Check sheet for the drawn part. Datum: minimum x, y, z corner. Units: mm. A direction names the side the tool comes from. Give positions to 0.01 mm unless a question says otherwise; leave off trailing zeros. Order: outer loops, then holes, each group sorted by start corner. A loop starts at its lowest first (then second) coordinate and runs counter-clockwise, first axis right, second up. Notation, with made-up numbers: (73.5, 21) - (114.5, 21) arc R27 ccw to (114.5, 57) - close; hole circle Ø2 at (46.25, 85.25). An arc over 180 degrees is marked (long way). Answer as a JSON object with one key per item and string values. Group by question number.
(1) Depth check by flat-ended pin: pin 1 Ø4.5 at (x, y) = (19.5, 3) entering from -Z; pin 2 Ø1.5 at (x, z) = (13, 29) entering from +Y; pin 3 Ø1 at (y, z) = (1, 24.5) entering from +X. Enter the tip coordinate at first touch or a pass-through.
(2) Section check B-B (x = 7.5). Record the boundary of the cut face in (y, z), then the cut area to 3 significant figures.
(3) Access from +Z, -Z, +X, -X, +Y, -Y to the whole of each face (thin tool, end or side, straight path). Record for the marked faces 4, 5 and 6.
(4) Thickness scan on line 1 (Z direction, x = 7.5, y = 0.95); line 2 (X direction, y = 1.45, z = 8); line 3 (Z direction, x = 16.75, y = 7). Record the ranges inside material, lowest first.
(5) Mould release check, pull along Z, two halves, no side actions. Record for the marked faces 1, 2 and 3: +Z half, -Z half, draft (parallel to the pull), parting line (faces both ways), or undercut.
(6) Section check A-A (z = 33). Record the boundary of the cut face in (x, y), then the cut area to 3 significant figures.
(7) Section check C-C (y = 8.5). Record the boundary of the cut face in (x, z).
(8) Section check D-D (z = 15). Record the boundary of the cut face in (x, y).
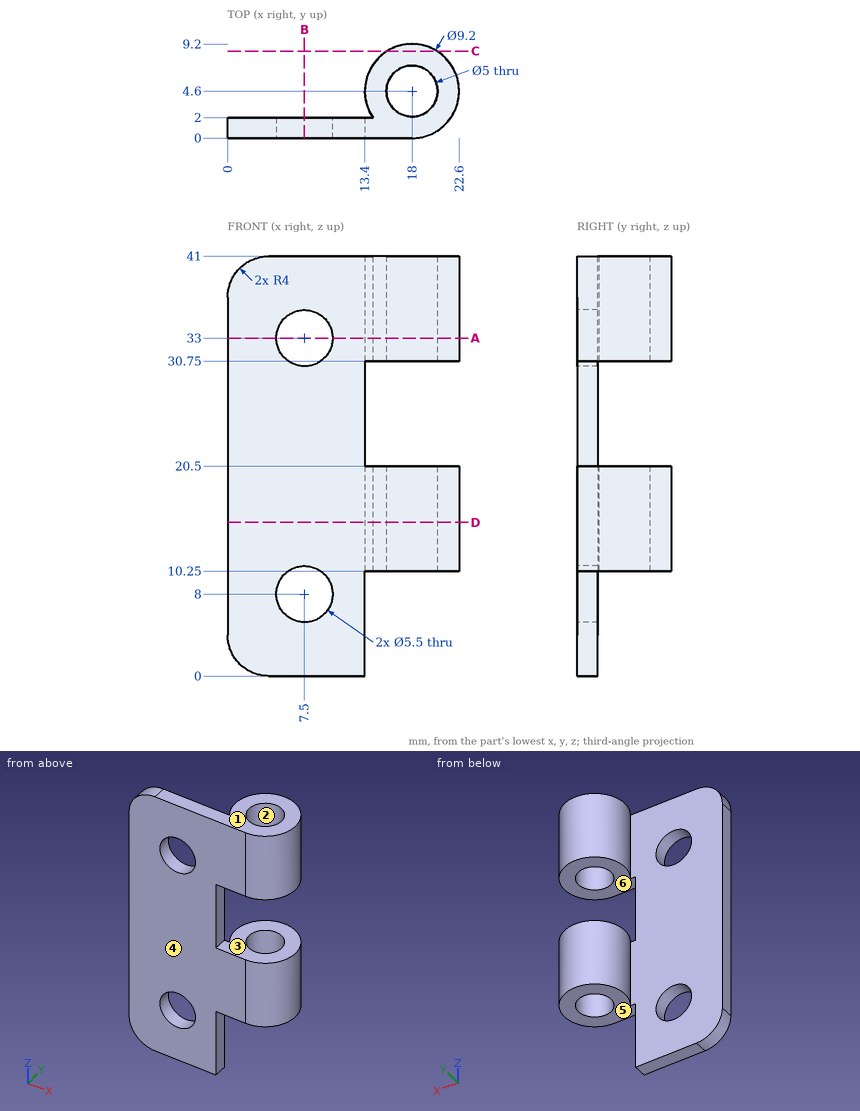
Solutions:
{
 "1": {"pin 1": "stops at z = 10.25", "pin 2": "stops at y = 2", "pin 3": "stops at x = 13.4"},
 "2": {"outline": "(0, 0) - (2, 0) - (2, 5.25) - (0, 5.25) - close; (0, 10.75) - (2, 10.75) - (2, 30.25) - (0, 30.25) - close; (0, 35.75) - (2, 35.75) - (2, 41) - (0, 41) - close", "area": "60.0 mm2"},
 "3": {"face 4": "+Z, -Z, +X, -X, -Y", "face 5": "-Z, +X, +Y, -Y", "face 6": "+X, +Y, -Y"},
 "4": {"line 1": "z = 0 to 5.25, 10.75 to 30.25, 35.75 to 41", "line 2": "x = 0 to 4.75, 10.25 to 13.4", "line 3": "z = 10.25 to 20.5, 30.75 to 41"},
 "5": {"face 1": "+Z half", "face 2": "draft", "face 3": "undercut"},
 "6": {"outline": "(0, 0) - (4.75, 0) - (4.75, 2) - (0, 2) - close; (10.25, 0) - (18, 0) arc R4.6 ccw (long way) to (14.21, 2) - (10.25, 2) - close; hole circle Ø5 at (18, 4.6)", "area": "66.5 mm2"},
 "7": {"outline": "(15.56, 10.25) - (20.44, 10.25) - (20.44, 20.5) - (15.56, 20.5) - close; (15.56, 30.75) - (20.44, 30.75) - (20.44, 41) - (15.56, 41) - close"},
 "8": {"outline": "(0, 0) - (18, 0) arc R4.6 ccw (long way) to (14.21, 2) - (0, 2) - close; hole circle Ø5 at (18, 4.6)"}
}
